from build123d import *

# Parameters (mm, degrees)
F1_DEPTH = 25
F2_R     = 10
F2_R_2   = 5
F3_DEPTH = 25
F4_R     = 4.9411574471
F5_DEPTH = 25.001


with BuildPart() as f1:
    # F0 (on Top) → F1 (new body)
    with BuildSketch(Plane.XY):
        with BuildLine():
            Line((-20, -10), (20, -10))
            Line((20, -10), (20, 10))
            Line((20, 10), (-20, 10))
            ThreePointArc((-20, 10), (-12.9289321881, 7.0710678119), (-10, 0))
            ThreePointArc((-10, 0), (-12.9289321881, -7.0710678119), (-20, -10))
        make_face()
        with BuildLine():
            ThreePointArc((-20, 10), (-30, 0), (-20, -10))
            Line((-20, -10), (-20, -5))
            ThreePointArc((-20, -5), (-25, 0), (-20, 5))
            Line((-20, 5), (-20, 10))
        make_face()
        with BuildLine():
            Line((-20, -5), (-20, -10))
            ThreePointArc((-20, -10), (-12.9289321881, -7.0710678119), (-10, 0))
            ThreePointArc((-10, 0), (-12.9289321881, 7.0710678119), (-20, 10))
            Line((-20, 10), (-20, 5))
            ThreePointArc((-20, 5), (-16.4644660941, 3.5355339059), (-15, 0))
            ThreePointArc((-15, 0), (-16.4644660941, -3.5355339059), (-20, -5))
        make_face()
    extrude(amount=F1_DEPTH)

    # F2 (on face) → F3 (join)
    with BuildSketch(Plane.XY.offset(25)):
        with Locations((20, 0)):
            Circle(F2_R)
        with Locations((20, 0)):
            Circle(F2_R_2, mode=Mode.SUBTRACT)
    extrude(amount=-F3_DEPTH)

    # F4 (on face) → F5 (cut, through all)
    with BuildSketch(Plane.XY.offset(25)):
        with Locations((20, 0)):
            Circle(F4_R)
    extrude(amount=-F5_DEPTH, mode=Mode.SUBTRACT)


solid = f1.part
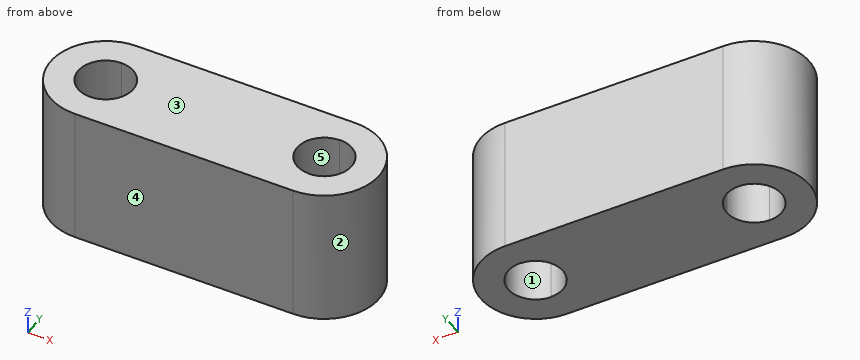
Design review of the part built by this model. Coordinates are the model's own, in mm. Face numbers are marked on the shaded views. A direction names the side the tool comes from. Coordinates: 2 decimals unless noted, no trailing zeros. Loops run counter-clockwise (first coordinate to the right, second up) from the corner with the lowest first, then second, coordinate; pieces in that order, holes last.
Item 1: For the marked faces 1 and 2, list the 3-axis set-ups (+Z, -Z, +X, -X, +Y, -Y) from which the entire face can be reached by the end or side of a thin tool; tool diameter is ignored.
Completed:
face 1: +Z, -Z
face 2: +Z, -Z, +X
Item 2: Add section A-A (z = 12). Write out the cut boundary in (x, y).
Completed:
outline: (-20, -10) - (20, -10) arc R10 ccw to (20, 10) - (-20, 10) arc R10 ccw to start; hole circle Ø10 at (-20, 0); hole (20, -5) arc R5 ccw to (20, 5) - (20, 4.94) arc R4.94 ccw to (20, -4.94) - close
Item 3: Draft analysis for pull direction Y (two halves, no side actions). For the marked faces 3, 4 and 5, state which applies: pulls with the +Y half, pulls with the -Y half, needs draft (parallel to the pull), parting line crosses it, or undercut.
Completed:
face 3: needs draft
face 4: pulls with the -Y half
face 5: undercut
Item 4: Add section C-C (y = 1). Write out the cut boundary in (x, z).
Completed:
outline: (-29.95, 0) - (-24.9, 0) - (-24.9, 25) - (-29.95, 25) - close; (-15.1, 0) - (15.16, 0) - (15.16, 25) - (-15.1, 25) - close; (24.9, 0) - (29.95, 0) - (29.95, 25) - (24.9, 25) - close
Item 5: Wall thickness on L1, parallel to X at y = -0.25, z = 20.25; L2, parallel to X at y = -4.5, z = 19; L3, parallel to Y at x = 24, z = 3.5: over which ranges is each line inside the solid? List them lowest first.
Completed:
L1: x = -30 to -24.99, -15.01 to 15.07, 24.99 to 30
L2: x = -28.93 to -22.18, -17.82 to 17.96, 22.18 to 28.93
L3: y = -9.17 to -3, 3 to 9.17
Item 6: Add section B-B (y = -1.5). Write out the cut boundary in (x, z).
Completed:
outline: (-29.89, 0) - (-24.77, 0) - (-24.77, 25) - (-29.89, 25) - close; (-15.23, 0) - (15.29, 0) - (15.29, 25) - (-15.23, 25) - close; (24.77, 0) - (29.89, 0) - (29.89, 25) - (24.77, 25) - close
Item 7: Add section D-D (y = 6.25). Write out the cut boundary in (x, z), and give its area (3 significant figures).
Completed:
outline: (-27.81, 0) - (27.81, 0) - (27.81, 25) - (-27.81, 25) - close
area: 1,390 mm2
Item 8: Clearance check with flat-ended pins moving along their axes: pin 1 (5 mm diameter, centred on y = 4.5, z = 16.5, fed in from +X); pin 2 (3 mm diameter, centred on y = 6.5, z = 12, fed in from -X); pin 3 (1.5 mm diameter, centred on y = 1, z = 20.5, fed in from +X). State where each tip first meets the part, or that it passes through.
Completed:
pin 1: stops at x = 29.8
pin 2: stops at x = -28.66
pin 3: stops at x = 30
